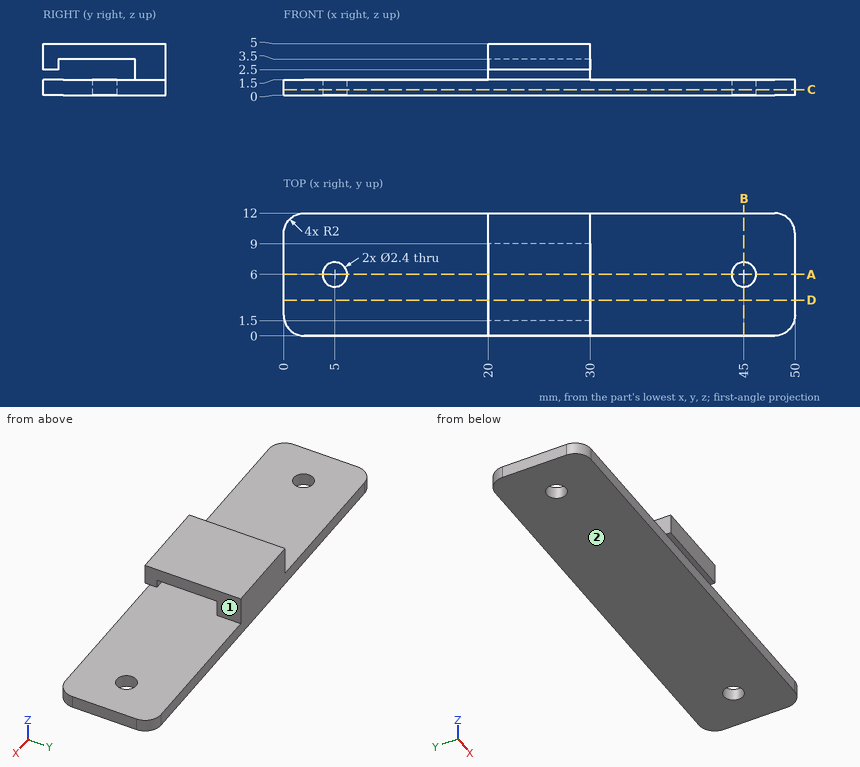
Part print with two shaded views. Sizes in mm from the minimum x, y, z corner. A direction names the side the tool comes from. Coordinates: 2 decimals unless noted, no trailing zeros. Write each loop counter-clockwise with the first axis right and the second up, starting at its lowest first coordinate (ties: lowest second). Pieces come first, ordered by that corner, then holes.
(1) Cut at B-B on x = 45. List the corners of the cut face in (y, z), and give its area (3 significant figures).
(2) Cut at A-A on y = 6. List the corners of the cut face in (x, z).
(3) Pin check, flat tips, straight feed: pin 1 Ø1.8 at (y, z) = (6.5, 4) entering from +X; pin 2 Ø1.4 at (x, y) = (5, 6) entering from -Z; pin 3 Ø1.8 at (y, z) = (5.5, 4) entering from -X. Stop position of each tip, or through.
(4) Cut at C-C on z = 0.55. List the corners of the cut face in (x, y).
(5) Drill centre lines: line 1 (Z direction, x = 23, y = 1); line 2 (Y direction, x = 45, z = 1.05); line 3 (Z direction, x = 25.5, y = 7). Where is each one in solid material? Low to high.
(6) 3-axis set-ups, long thin cutter, end or side, ignore diameter. For the marked faces 1 and 2: which of +Z, -Z, +X, -X, +Y, -Y reach the whole face in a straight line?
(7) Cut at D-D on y = 3.5. List the corners of the cut face in (x, z), and give its area (3 significant figures).
Working result:
1. outline: (0, 0) - (4.8, 0) - (4.8, 1.5) - (0, 1.5) - close; (7.2, 0) - (12, 0) - (12, 1.5) - (7.2, 1.5) - close
1. area: 14.4 mm2
2. outline: (0, 0) - (3.8, 0) - (3.8, 1.5) - (0, 1.5) - close; (6.2, 0) - (43.8, 0) - (43.8, 1.5) - (6.2, 1.5) - close; (20, 3.5) - (30, 3.5) - (30, 5) - (20, 5) - close; (46.2, 0) - (50, 0) - (50, 1.5) - (46.2, 1.5) - close
3. pin 1: stops at x = 30
3. pin 2: passes through
3. pin 3: stops at x = 20
4. outline: (0, 2) arc R2 ccw to (2, 0) - (48, 0) arc R2 ccw to (50, 2) - (50, 10) arc R2 ccw to (48, 12) - (2, 12) arc R2 ccw to (0, 10) - close; hole circle Ø2.4 at (5, 6); hole circle Ø2.4 at (45, 6)
5. line 1: z = 0 to 1.5, 2.5 to 5
5. line 2: y = 0 to 4.8, 7.2 to 12
5. line 3: z = 0 to 1.5, 3.5 to 5
6. face 1: +Z, +X, +Y, -Y
6. face 2: -Z, +X, -X, +Y, -Y
7. outline: (0, 0) - (50, 0) - (50, 1.5) - (0, 1.5) - close; (20, 3.5) - (30, 3.5) - (30, 5) - (20, 5) - close
7. area: 90.0 mm2
